The figure shows three views and two pictorial views of one solid part (mm, origin at its lowest corner). Answer the questions. A direction names the side the tool comes from. Give positions to 0.01 mm unless a question says otherwise; leave off trailing zeros. Loops run counter-clockwise (first coordinate to the right, second up) from the corner with the lowest first, then second, coordinate; pieces in that order, holes last. Notation, with made-up numbers: (53.5, 33) - (92.5, 33) arc R21 ccw to (92.5, 46) - close; hole circle Ø3 at (70.25, -27). An arc over 180 degrees is marked (long way). One line per question, with ' | ' between items.
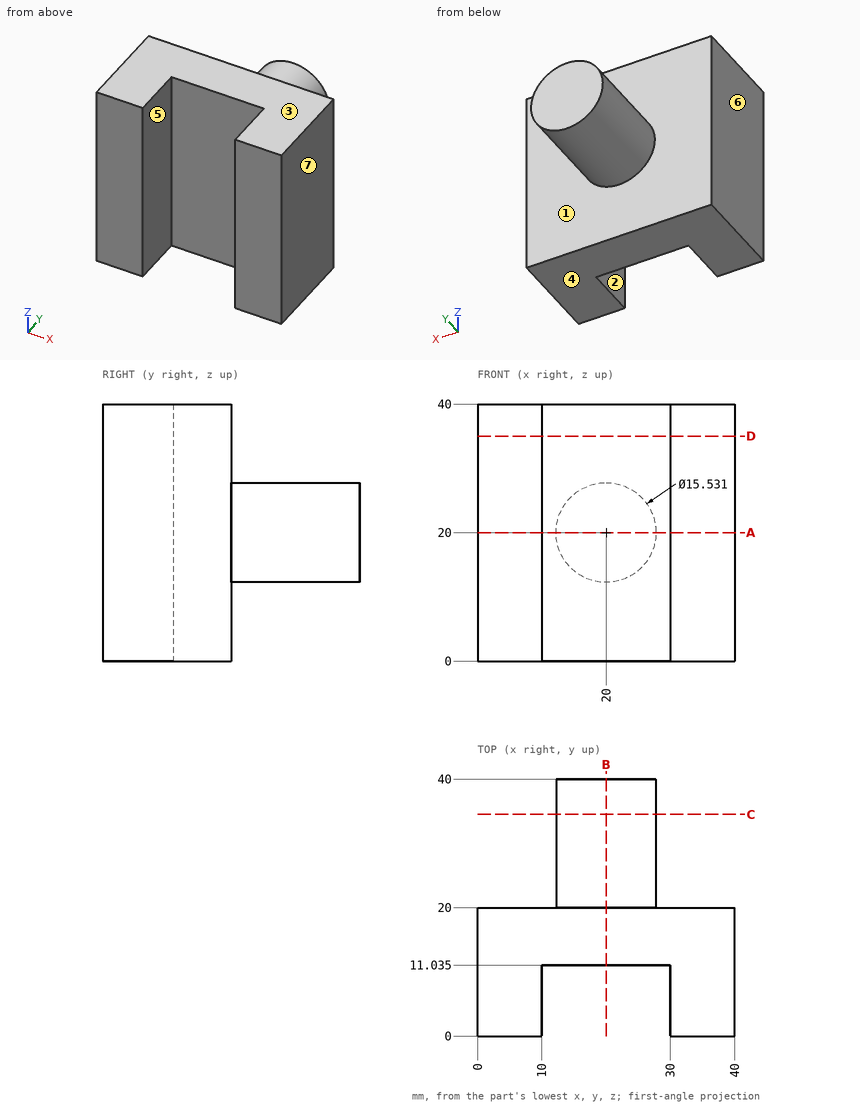
1. Consider L1, parallel to X at y = 11, z = 3; L2, parallel to Y at x = 24, z = 6.5 (1 decimal); L3, parallel to Y at x = 37.5, z = 3. Determine where each line is inside the solid, lowest interval first.
Evaluation:
L1: 0 to 10, 30 to 40 | L2: 11 to 20 | L3: 0 to 20
2. Which of the six approach directions +Z, -Z, +X, -X, +Y, -Y give full straight-line access (tool end or side, diameter ignored) to the marked faces 1, 2 and 3?
Evaluation:
face 1: +Y | face 2: +Z, -Z, -Y | face 3: +Z, +X, -X, +Y, -Y
3. Find section D-D on z = 35. Write down the section's boundary in (x, y) (1 decimal), then the cut area to 3 significant figures.
Evaluation:
outline: (0, 0) - (10, 0) - (10, 11) - (30, 11) - (30, 0) - (40, 0) - (40, 20) - (0, 20) - close | area: 579 mm2
4. Find section C-C on y = 34.5. Write down the section's boundary in (x, z) (1 decimal), then the cut area to 3 significant figures.
Evaluation:
outline: circle Ø15.5 at (20, 20) | area: 189 mm2
5. Find section B-B on x = 20. Write down the section's boundary in (y, z) (1 decimal), then the cut area to 3 significant figures.
Evaluation:
outline: (11, 0) - (20, 0) - (20, 12.2) - (40, 12.2) - (40, 27.8) - (20, 27.8) - (20, 40) - (11, 40) - close | area: 669 mm2
6. Determine the mould class of the marked faces 4, 5, 6 and 7 for opening direction X: +X half, -X half, draft (parallel to the pull), parting line (faces both ways), or undercut.
Evaluation:
face 4: draft | face 5: undercut | face 6: -X half | face 7: +X half
7. Find section A-A on z = 20. Write down the section's boundary in (x, y) (1 decimal), then the cut area to 3 significant figures.
Evaluation:
outline: (0, 0) - (10, 0) - (10, 11) - (30, 11) - (30, 0) - (40, 0) - (40, 20) - (27.8, 20) - (27.8, 40) - (12.2, 40) - (12.2, 20) - (0, 20) - close | area: 890 mm2
8. Flat-ended cylindrical pins translate along their axes: pin 1 (2 mm diameter, centred on x = 5.5, z = 5.5, fed in from +Y); pin 2 (1 mm diameter, centred on x = 15.5, y = 35, fed in from -Z) (1 decimal); pin 3 (10 mm diameter, centred on x = 16.5, z = 18, fed in from -Y) (1 decimal). Find the tip coordinate at first contact, or state that the pin passes through.
Evaluation:
pin 1: y = 20 | pin 2: z = 13.3 | pin 3: y = 11
